Could you check a few things on this drawing? It's one solid part, dimensions in mm from its lowest x, y, z. Give positions to 0.01 mm unless a question says otherwise; leave off trailing zeros. Loops run counter-clockwise (first coordinate to the right, second up) from the corner with the lowest first, then second, coordinate; pieces in that order, holes last. Notation, with made-up numbers: M 0,-33.75 L 36,-33.75 A21 ccw 36,-16.75 Z; hole C 89,-15.75 d8. An arc over 180 degrees is marked long. Answer as a JSON object with one key per item and string values.
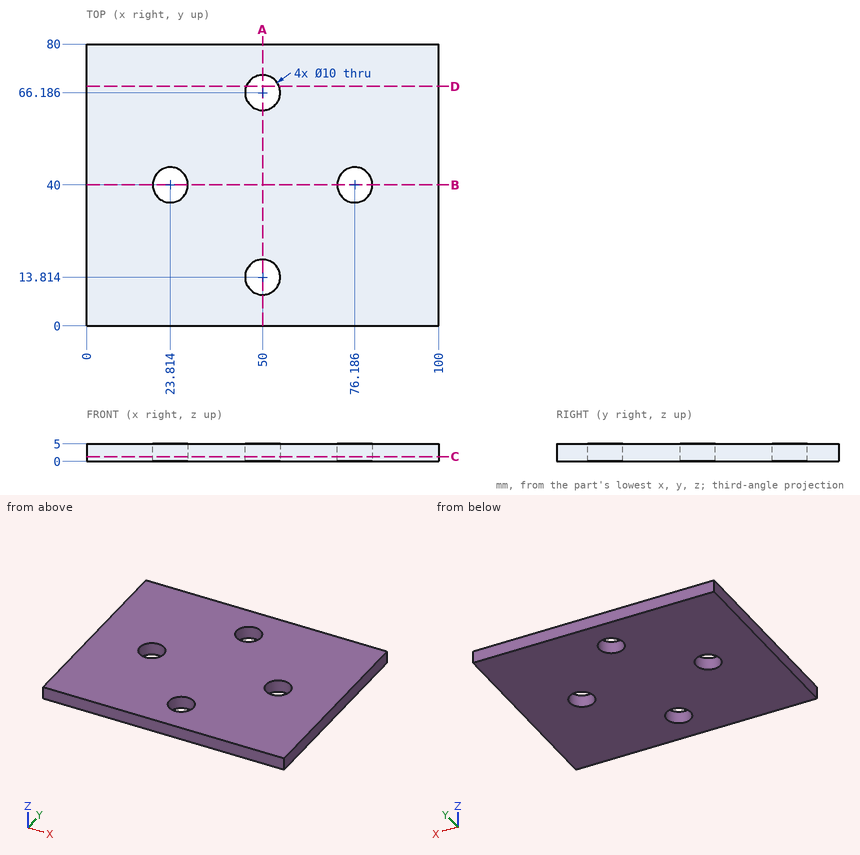
1) Will this pin go through, and if not, where does the flat tip stop? pin 1 Ø8 at (x, y) = (76.19, 40) entering from +Z.
Answer list:
{"pin 1": "through"}
2) Please list where these lines run through material, in increasing order: line 1 along Y through (x, z) = (50, 3.65); line 2 along X through (y, z) = (42, 3.2); line 3 along X through (y, z) = (15, 2.35). Write a range as from..to.
Answer list:
{"line 1": "0..8.81, 18.81..61.19, 71.19..80", "line 2": "0..19.23, 28.4..71.6, 80.77..100", "line 3": "0..45.14, 54.86..100"}
3) Suppose I cut it at A-A, the plane x = 50. Write out the boundary of the cut face in (y, z).
Answer list:
{"outline": "M 0,0 L 8.81,0 L 8.81,5 L 0,5 Z; M 18.81,0 L 61.19,0 L 61.19,5 L 18.81,5 Z; M 71.19,0 L 80,0 L 80,5 L 71.19,5 Z"}
4) Suppose I cut it at C-C, the plane z = 1.35. Write out the boundary of the cut face in (x, y), and give its area (3 significant figures).
Answer list:
{"outline": "M 0,0 L 100,0 L 100,80 L 0,80 Z; hole C 23.81,40 d10; hole C 50,13.81 d10; hole C 50,66.19 d10; hole C 76.19,40 d10", "area": "7,690 mm^2"}
5) Suppose I cut it at D-D, the plane y = 68. Write out the boundary of the cut face in (x, z).
Answer list:
{"outline": "M 0,0 L 45.34,0 L 45.34,5 L 0,5 Z; M 54.66,0 L 100,0 L 100,5 L 54.66,5 Z"}
6) Suppose I cut it at B-B, the plane y = 40. Write out the boundary of the cut face in (x, z).
Answer list:
{"outline": "M 0,0 L 18.81,0 L 18.81,5 L 0,5 Z; M 28.81,0 L 71.19,0 L 71.19,5 L 28.81,5 Z; M 81.19,0 L 100,0 L 100,5 L 81.19,5 Z"}
